Check sheet for the drawn part. Datum: minimum x, y, z corner. Units: mm. A direction names the side the tool comes from. Coordinates: 2 decimals unless noted, no trailing zeros. Order: outer loops, then holes, each group sorted by start corner. A loop starts at its lowest first (then second) coordinate and runs counter-clockwise, first axis right, second up.
Q1. Draft check along Z on the marked faces 3, 4 and 5. Enter one of: pulls with the +Z half, pulls with the -Z half, needs draft (parallel to the pull), parting line crosses it, or undercut.
Q2. Cross-section at D-D, the plane y = 1.5. Record the boundary of the cut face in (x, z) (1 decimal).
Q3. Thickness scan on line 1 (Z direction, x = 2.5, y = 5.5); line 2 (Y direction, x = 7.75, z = 12.5) (1 decimal); line 3 (Y direction, x = 11, z = 17) (1 decimal). Record the ranges inside material, lowest first.
Q4. Cross-section at B-B, the plane x = 5.5. Record the boundary of the cut face in (y, z).
Q5. Cross-section at A-A, the plane y = 13.5. Record the boundary of the cut face in (x, z) (1 decimal).
Q6. Depth check by flat-ended pin: P1, Ø4, axis at x = 4.5, z = 15, coming from the -Y side; P2, Ø1, axis at x = 9.5, z = 24, coming from the -Y side; P3, Ø1, axis at x = 9.5, z = 10, coming from the +Y side. Enter the tip coordinate at first touch or a pass-through.
Q7. Set-up check for the marked faces 1 and 2: record each of +Z, -Z, +X, -X, +Y, -Y from which the full face is reachable in a straight line by a thin tool's end or side.
Q8. Cross-section at C-C, the plane y = 5.25. Record the boundary of the cut face in (x, z), and give its area (3 significant figures).
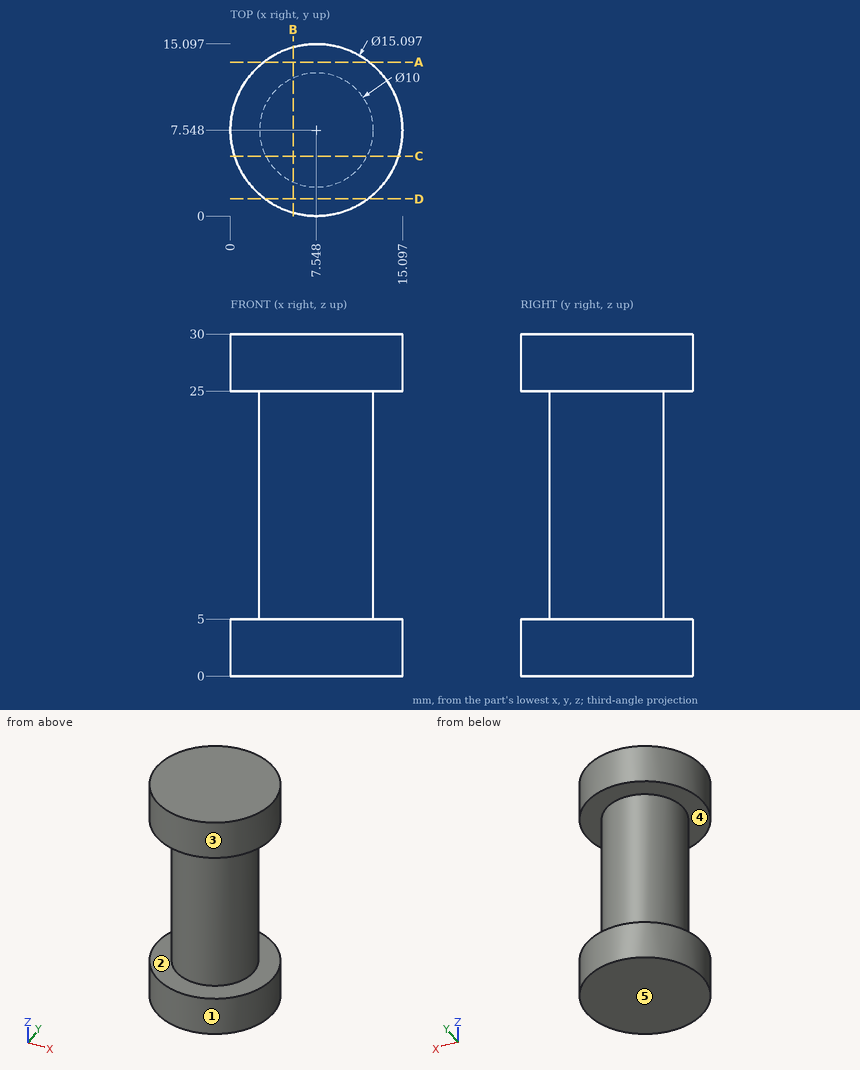
Check values:
1. face 3: needs draft
1. face 4: undercut
1. face 5: pulls with the -Z half
2. outline: (3, 0) - (12.1, 0) - (12.1, 5) - (3, 5) - close; (3, 25) - (12.1, 25) - (12.1, 30) - (3, 30) - close
3. line 1: z = 0 to 5, 25 to 30
3. line 2: y = 2.6 to 12.5
3. line 3: y = 3.9 to 11.2
4. outline: (0.28, 0) - (14.81, 0) - (14.81, 5) - (12.11, 5) - (12.11, 25) - (14.81, 25) - (14.81, 30) - (0.28, 30) - (0.28, 25) - (2.99, 25) - (2.99, 5) - (0.28, 5) - close
5. outline: (2.9, 0) - (12.2, 0) - (12.2, 5) - (2.9, 5) - close; (2.9, 25) - (12.2, 25) - (12.2, 30) - (2.9, 30) - close
6. P1: stops at y = 2.66
6. P2: stops at y = 2.76
6. P3: stops at y = 12.33
7. face 1: +Z, -Z
7. face 2: none
8. outline: (0.36, 0) - (14.74, 0) - (14.74, 5) - (11.99, 5) - (11.99, 25) - (14.74, 25) - (14.74, 30) - (0.36, 30) - (0.36, 25) - (3.11, 25) - (3.11, 5) - (0.36, 5) - close
8. area: 321 mm2
